Verification items for the finished model (mm, model axes). A direction names the side the tool comes from. Coordinates: 2 decimals unless noted, no trailing zeros. Write each loop counter-clockwise with the first axis right and the second up, starting at its lowest first coordinate (ties: lowest second). Pieces come first, ordered by that corner, then holes. Notation, with made-up numbers: M 9,57.5 L 21,57.5 A16 cw 21,73.5 Z; hole C 67.5,-36 d8. An arc over 180 degrees is marked long. Answer in a Markdown table with one row per item.
from build123d import *

# Parameters (mm, degrees)
CIRCULARBAND_W               = 15
CIRCULARBAND_H               = 0.75
BASE_REVOLVE_ANGLE           = 120
BASE_REVOLVE_OTHER_WAY_ANGLE = 120
SKETCH9_OUTSIDE_W            = 25.428
SKETCH9_OUTSIDE_H            = 34.053
HEAD1_DEPTH                  = 16.75
SKETCH10_OUTSIDE_W           = 25.428
SKETCH10_OUTSIDE_H           = 34.053
TAIL1_DEPTH                  = 16.75


with BuildPart() as part:
    # circularband → Base-Revolve (revolve)
    with BuildSketch(Plane.XY):
        with Locations((0, 15.375)):
            Rectangle(CIRCULARBAND_W, CIRCULARBAND_H)
    revolve(axis=Axis((0, 0, 0), (1, 0, 0)), revolution_arc=BASE_REVOLVE_ANGLE)

    # circularband → Base-Revolve other way (revolve)
    with BuildSketch(Plane.XY):
        with Locations((0, 15.375)):
            Rectangle(CIRCULARBAND_W, CIRCULARBAND_H)
    revolve(axis=Axis((0, 0, 0), (-1, 0, 0)), revolution_arc=BASE_REVOLVE_OTHER_WAY_ANGLE)

    # Sketch9 outside → head1 (cut, through all)
    with BuildSketch(Plane.XY):
        with Locations((0, 3.9375)):
            Rectangle(SKETCH9_OUTSIDE_W, SKETCH9_OUTSIDE_H)
        Polygon((-3.375, 15.75), (3.375, 15.75), (3.375, 6.490381057), (7.5, 6.490381057), (0, -6.5), (-7.5, 6.490381057), (-3.375, 6.490381057), align=None, mode=Mode.SUBTRACT)
    extrude(amount=-HEAD1_DEPTH, mode=Mode.SUBTRACT)

    # Sketch10 outside → tail1 (cut, through all)
    with BuildSketch(Plane.XY):
        with Locations((0, 3.9375)):
            Rectangle(SKETCH10_OUTSIDE_W, SKETCH10_OUTSIDE_H)
        Polygon((0, -2.029328524), (3.375, -7.875), (3.375, 15.75), (-3.375, 15.75), (-3.375, -7.875), align=None, mode=Mode.SUBTRACT)
    extrude(amount=TAIL1_DEPTH, mode=Mode.SUBTRACT)


solid = part.part
1) Depth check by flat-ended pin: pin 1 (0.9 mm diameter, centred on x = -6, z = -14, fed in from +Y); pin 2 (2 mm diameter, centred on x = -5.5, y = 4.5, fed in from +Z); pin 3 (4 mm diameter, centred on x = -2.5, y = -2.5, fed in from +Z). Enter the tip coordinate at first touch or a pass-through.
Response values:
| item | result |
|---|---|
| pin 1 | stops at y = 6.49 |
| pin 2 | stops at z = -13.96 |
| pin 3 | stops at z = 15.74 |
2) Release check for a two-part mould opening along X. For faces 1 (the face through (-5, 6.49, -14)), 2 (the face through (1.68, -4.94, 14.49)), 3 (the face through (-1.7, -4.97, 14.49)), 4 (the face through (3.375, 14.4, 5.1)) record: +X half, -X half, draft (parallel to the pull), parting line (faces both ways), or undercut.
Response values:
| item | result |
|---|---|
| face 1 | draft |
| face 2 | undercut |
| face 3 | undercut |
| face 4 | +X half |
3) Thickness scan on L1, parallel to Z at x = 0, y = 0; L2, parallel to Y at x = 0.5, z = 0; L3, parallel to X at y = 8, z = 13.5 (3 decimals). Record the ranges inside material, lowest first. Write a range as [from, to].
Response values:
| item | result |
|---|---|
| L1 | z = [-15.75, -15], [15, 15.75] |
| L2 | y = [15, 15.75] |
| L3 | x = [-3.375, 3.375] |
4) Sectioned sample at C-C (z = 10). Record the cut outline in (x, y) (3 decimals).
Response values:
| item | result |
|---|---|
| outline | M -3.375,11.18 L 3.375,11.18 L 3.375,12.168 L -3.375,12.168 Z |
5) Sectioned sample at B-B (y = -5.5). Record the cut outline in (x, z) (3 decimals).
Response values:
| item | result |
|---|---|
| outline | M -3.375,13.955 L -2.004,13.955 L -2.004,14.758 L -3.375,14.758 Z; M -0.577,-14.758 L 0.577,-14.758 L 0.577,-13.955 L -0.577,-13.955 Z; M 2.004,13.955 L 3.375,13.955 L 3.375,14.758 L 2.004,14.758 Z |
6) Sectioned sample at A-A (y = 11.75). Record the cut outline in (x, z) (3 decimals), then the cut area to 3 significant figures.
Response values:
| item | result |
|---|---|
| outline | M -3.375,-10.488 L 3.375,-10.488 L 3.375,-9.324 L -3.375,-9.324 Z; M -3.375,9.324 L 3.375,9.324 L 3.375,10.488 L -3.375,10.488 Z |
| area | 15.7 mm² |
7) Tool access check on faces 5 (the face through (5, 6.49, -14)), 6 (the face through (-3.73, -0.04, -15.37)), 7 (the face through (3.77, 0.03, -15.37)). Record the directions out of +Z, -Z, +X, -X, +Y, -Y that give a thin tool (end or side, any length) a straight path to the whole face; none if there is none.
Response values:
| item | result |
|---|---|
| face 5 | +Z, -Z, +X, +Y |
| face 6 | -Z, -X, -Y |
| face 7 | -Z, +X, -Y |
8) Sectioned sample at D-D (y = 0). Record the cut outline in (x, z) (3 decimals), then the cut area to 3 significant figures.
Response values:
| item | result |
|---|---|
| outline | M -3.753,-15.75 L 3.753,-15.75 L 3.753,-15 L -3.753,-15 Z; M -3.375,15 L 3.375,15 L 3.375,15.75 L -3.375,15.75 Z |
| area | 10.7 mm² |
